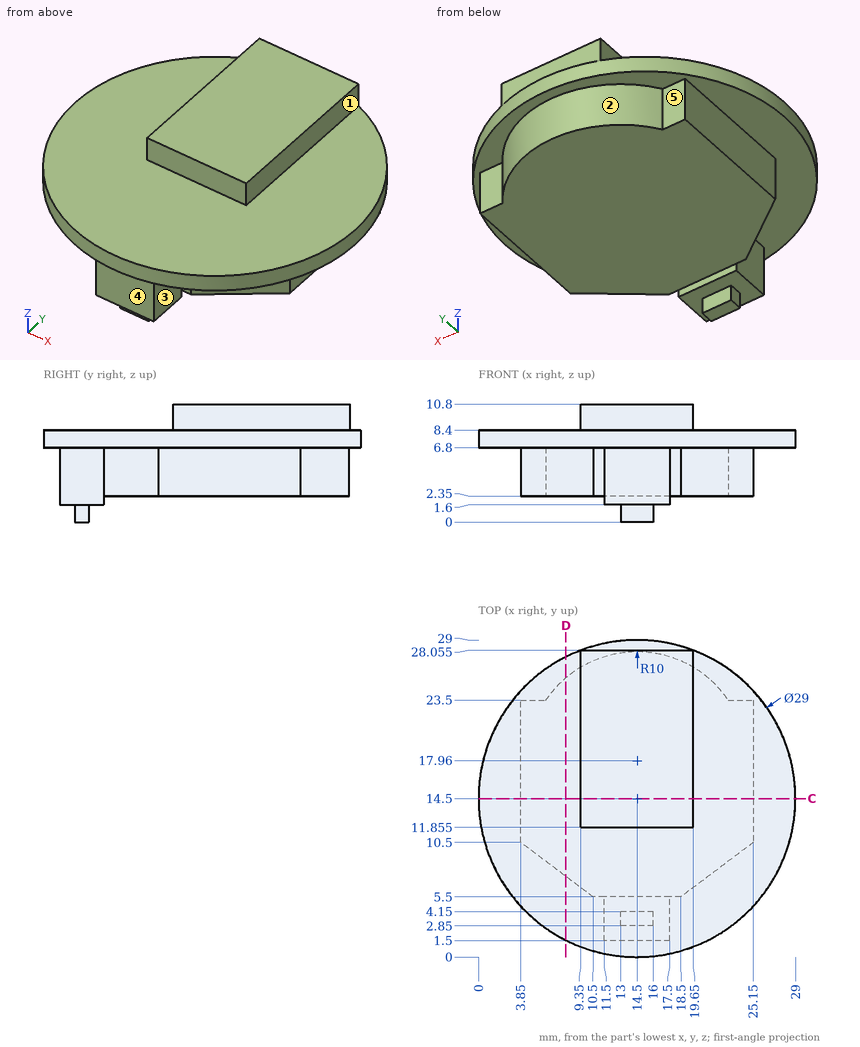
Input: dimensioned drawing with shaded views. Units: mm. Origin: part minimum x, y, z. A direction names the side the tool comes from. Round coordinates to 2 decimals unless told otherwise and drop trailing zeros. Loops run counter-clockwise (first coordinate to the right, second up) from the corner with the lowest first, then second, coordinate; pieces in that order, holes last. Notation, with made-up numbers: (51.5, 40) -> (84.5, 40) arc R22 ccw to (84.5, 79) -> close; hole circle Ø3 at (-3.75, 20). An arc over 180 degrees is marked (long way). Answer as a JSON object with one key per item and string values. Group by question number.
Q1. Ray query, line 1 (Z direction, x = 26, y = 23.25); line 2 (Z direction, x = 14.5, y = 8.75); line 3 (Y direction, x = 19, z = 10.25) (1 decimal). Return the intervals inside material, ascending. Write a range as from..to.
Q2. Contact query for flat-ended pins moving along their axis: P1, Ø3, axis at x = 7.5, y = 15.5, coming from the +Z side; P2, Ø8.5, axis at x = 20.5, y = 8, coming from the -Z side; P3, Ø1, axis at y = 17, z = 6, coming from the +X side; P4, Ø4.5, axis at x = 16, y = 3.5, coming from the -Z side. Output: stop coordinate, or through.
Q3. Section query D-D (x = 8). Output: boundary loops of the cut face in (y, z), plus the area to 3 significant figures.
Q4. Access query for the marked faces 1, 2, 3, 4 and 5. Directions: +Z, -Z, +X, -X, +Y, -Y. A direction counts if a zero-diameter tool reaches every point of the face in a straight line with its end or side. Return the directions, or none.
Q5. Section query C-C (y = 14.5). Output: boundary loops of the cut face in (x, z).
Completed:
{
 "1": {"line 1": "6.8..8.4", "line 2": "2.35..8.4", "line 3": "11.9..28.1"},
 "2": {"P1": "z = 8.4", "P2": "z = 1.6", "P3": "x = 25.15", "P4": "z = 0"},
 "3": {"outline": "(1.54, 6.8) -> (7.38, 6.8) -> (7.38, 2.35) -> (25.56, 2.35) -> (25.56, 6.8) -> (27.46, 6.8) -> (27.46, 8.4) -> (1.54, 8.4) -> close", "area": "122 mm²"},
 "4": {"face 1": "+Z, +X, +Y, -Y", "face 2": "-Z, +Y", "face 3": "-Z, +X, -Y", "face 4": "-Z, +X, -X, -Y", "face 5": "-Z, -X, +Y"},
 "5": {"outline": "(0, 6.8) -> (3.85, 6.8) -> (3.85, 2.35) -> (25.15, 2.35) -> (25.15, 6.8) -> (29, 6.8) -> (29, 8.4) -> (19.65, 8.4) -> (19.65, 10.8) -> (9.35, 10.8) -> (9.35, 8.4) -> (0, 8.4) -> close"}
}
